from build123d import *

# Parameters (mm, degrees)
SKIZZE2_W                        = 120
SKIZZE2_H                        = 39.364160046
AUFSATZ_LINEAR_AUSTRAGEN1_DEPTH  = 30
SKIZZE24_R                       = 1.55
SCHNITT_LINEAR_AUSTRAGEN4_DEPTH  = 130.805766806
SKIZZE46_R                       = 2.85
SCHNITT_LINEAR_AUSTRAGEN15_DEPTH = 10
SCHNITT_LINEAR_START             = -5
SCHNITT_LINEAR_AUSTRAGEN25_DEPTH = 2.7
LINEARES_MUSTER1_COUNT           = 4
LINEARES_MUSTER1_PITCH           = 20
SPIEGELN2_COPY_1_SKETCH_R        = 2.85
SPIEGELN2_COPY_1_DEPTH           = 10
SPIEGELN2_COPY_2_SKETCH_R        = 2.85
SPIEGELN2_COPY_2_DEPTH           = 10
SPIEGELN2_COPY_3_SKETCH_R        = 2.85
SPIEGELN2_COPY_3_DEPTH           = 10
SPIEGELN2_START                  = -5
SPIEGELN2_COPY_4_DEPTH           = 2.7
SPIEGELN2_COPY_5_DEPTH           = 2.7
SPIEGELN2_COPY_6_DEPTH           = 2.7
SKIZZE51_R                       = 1.55
SCHNITT_LINEAR_AUSTRAGEN26_DEPTH = 130.805766806
SKIZZE75_R                       = 0.75
SCHNITT_LINEAR_AUSTRAGEN28_DEPTH = 10
SKIZZE76_R                       = 2
SCHNITT_LINEAR_AUSTRAGEN29_DEPTH = 6
SKIZZE80_R                       = 0.5
SCHNITT_LINEAR_AUSTRAGEN34_DEPTH = 21
SCHNITT_LINEAR_START_2           = -7.5
SKIZZE81_R                       = 0.5
SCHNITT_LINEAR_AUSTRAGEN36_DEPTH = 5
ABSPALTEN3_START                 = 15
ABSPALTEN3_OUTLINE_W             = 120
ABSPALTEN3_OUTLINE_H             = 39.364160046
ABSPALTEN3_OUTLINE_R             = 1.55
ABSPALTEN3_DEPTH                 = 15


# Read off the part's stored shape, not the designer's step: Abspalten3
with BuildPart() as part:
    # Skizze2 → Aufsatz-Linear austragen1 (new body)
    with BuildSketch(Plane.XY):
        with Locations((60, 19.682080023)):
            Rectangle(SKIZZE2_W, SKIZZE2_H)
    extrude(amount=AUFSATZ_LINEAR_AUSTRAGEN1_DEPTH)

    # Skizze24 → Schnitt-Linear austragen4 (cut, through all)
    with BuildSketch(Plane.XY.offset(30)):
        with Locations((40, 31.364160046)):
            Circle(SKIZZE24_R)
        with Locations((60, 31.364160046)):
            Circle(SKIZZE24_R)
        with Locations((80, 31.364160046)):
            Circle(SKIZZE24_R)
        with Locations((100, 31.364160046)):
            Circle(SKIZZE24_R)
    schnitt_linear_austragen4 = extrude(amount=-SCHNITT_LINEAR_AUSTRAGEN4_DEPTH, mode=Mode.SUBTRACT)

    # Skizze46 → Schnitt-Linear austragen15 (cut)
    with BuildSketch(Plane(origin=(0, 0, 0), x_dir=(-1, 0, 0), z_dir=(0, 0, -1))):
        with Locations((-100, 31.364160046)):
            Circle(SKIZZE46_R)
    schnitt_linear_austragen15 = extrude(amount=-SCHNITT_LINEAR_AUSTRAGEN15_DEPTH, mode=Mode.SUBTRACT)

    # Skizze50 → Schnitt-Linear austragen25 (cut)
    with BuildSketch(Plane.XY.offset(30).offset(SCHNITT_LINEAR_START)):
        Polygon((97.15, 33.009608314), (97.15, 39.364160046), (102.85, 39.364160046), (102.85, 33.009608314), (102.85, 29.718711779), (100, 28.073263512), (97.15, 29.718711779), align=None)
    schnitt_linear_austragen25 = extrude(amount=-SCHNITT_LINEAR_AUSTRAGEN25_DEPTH, mode=Mode.SUBTRACT)

    # Lineares Muster1: Schnitt-Linear austragen15, Schnitt-Linear austragen25 ×4
    with Locations(*[(-i * LINEARES_MUSTER1_PITCH, 0, 0) for i in range(1, LINEARES_MUSTER1_COUNT)]):
        add(schnitt_linear_austragen15, mode=Mode.SUBTRACT)
        add(schnitt_linear_austragen25, mode=Mode.SUBTRACT)

    # Spiegeln2: Schnitt-Linear austragen15, Schnitt-Linear austragen25 across plane
    add(schnitt_linear_austragen15.mirror(Plane.ZX.offset(19.764160046)), mode=Mode.SUBTRACT)
    add(schnitt_linear_austragen25.mirror(Plane.ZX.offset(19.764160046)), mode=Mode.SUBTRACT)

    # Spiegeln2 copy 1 sketch → Spiegeln2 copy 1 (cut)
    with BuildSketch(Plane(origin=(-20, 39.528320093, 0), x_dir=(-1, 0, 0), z_dir=(0, 0, -1))):
        with Locations((-100, -31.364160046)):
            Circle(SPIEGELN2_COPY_1_SKETCH_R)
    extrude(amount=-SPIEGELN2_COPY_1_DEPTH, mode=Mode.SUBTRACT)

    # Spiegeln2 copy 2 sketch → Spiegeln2 copy 2 (cut)
    with BuildSketch(Plane(origin=(-40, 39.528320093, 0), x_dir=(-1, 0, 0), z_dir=(0, 0, -1))):
        with Locations((-100, -31.364160046)):
            Circle(SPIEGELN2_COPY_2_SKETCH_R)
    extrude(amount=-SPIEGELN2_COPY_2_DEPTH, mode=Mode.SUBTRACT)

    # Spiegeln2 copy 3 sketch → Spiegeln2 copy 3 (cut)
    with BuildSketch(Plane(origin=(-60, 39.528320093, 0), x_dir=(-1, 0, 0), z_dir=(0, 0, -1))):
        with Locations((-100, -31.364160046)):
            Circle(SPIEGELN2_COPY_3_SKETCH_R)
    extrude(amount=-SPIEGELN2_COPY_3_DEPTH, mode=Mode.SUBTRACT)

    # Spiegeln2 copy 4 sketch → Spiegeln2 copy 4 (cut)
    with BuildSketch(Plane(origin=(-20, 39.528320093, 30), x_dir=(1, 0, 0), z_dir=(0, 0, 1)).offset(SPIEGELN2_START)):
        Polygon((97.15, -33.009608314), (97.15, -39.364160046), (102.85, -39.364160046), (102.85, -33.009608314), (102.85, -29.718711779), (100, -28.073263512), (97.15, -29.718711779), align=None)
    extrude(amount=-SPIEGELN2_COPY_4_DEPTH, mode=Mode.SUBTRACT)

    # Spiegeln2 copy 5 sketch → Spiegeln2 copy 5 (cut)
    with BuildSketch(Plane(origin=(-40, 39.528320093, 30), x_dir=(1, 0, 0), z_dir=(0, 0, 1)).offset(SPIEGELN2_START)):
        Polygon((97.15, -33.009608314), (97.15, -39.364160046), (102.85, -39.364160046), (102.85, -33.009608314), (102.85, -29.718711779), (100, -28.073263512), (97.15, -29.718711779), align=None)
    extrude(amount=-SPIEGELN2_COPY_5_DEPTH, mode=Mode.SUBTRACT)

    # Spiegeln2 copy 6 sketch → Spiegeln2 copy 6 (cut)
    with BuildSketch(Plane(origin=(-60, 39.528320093, 30), x_dir=(1, 0, 0), z_dir=(0, 0, 1)).offset(SPIEGELN2_START)):
        Polygon((97.15, -33.009608314), (97.15, -39.364160046), (102.85, -39.364160046), (102.85, -33.009608314), (102.85, -29.718711779), (100, -28.073263512), (97.15, -29.718711779), align=None)
    extrude(amount=-SPIEGELN2_COPY_6_DEPTH, mode=Mode.SUBTRACT)

    # Spiegeln3: Schnitt-Linear austragen4 across plane
    add(schnitt_linear_austragen4.mirror(Plane.ZX.offset(19.764160046)), mode=Mode.SUBTRACT)

    # Skizze51 → Schnitt-Linear austragen26 (cut, through all)
    with BuildSketch(Plane.XY.offset(30)):
        with Locations((5, 34.364160046)):
            Circle(SKIZZE51_R)
        with Locations((115, 5)):
            Circle(SKIZZE51_R)
    extrude(amount=-SCHNITT_LINEAR_AUSTRAGEN26_DEPTH, mode=Mode.SUBTRACT)

    # Skizze73 → Schnitt-Rotation5 (revolve, cut)
    with BuildSketch(Plane.XY.offset(15)):
        Polygon((15, 19.764160046), (15, 23.264160046), (20, 23.264160046), (20, 24.264160046), (100, 22.682080023), (100, 21.682080023), (105, 21.682080023), (105, 19.682080023), align=None)
    revolve(axis=Axis((105, 19.682080023, 15), (-0.9999995841280241, 0.0009119998787298228, 0)), mode=Mode.SUBTRACT)

    # Skizze75 → Schnitt-Linear austragen28 (cut)
    with BuildSketch(Plane.XY.offset(30)):
        with Locations((21.598259807, 19.682080023)):
            Circle(SKIZZE75_R)
    extrude(amount=-SCHNITT_LINEAR_AUSTRAGEN28_DEPTH, mode=Mode.SUBTRACT)

    # Skizze76 → Schnitt-Linear austragen29 (cut)
    with BuildSketch(Plane.XY.offset(30)):
        with Locations((21.598259807, 19.682080023)):
            Circle(SKIZZE76_R)
    extrude(amount=-SCHNITT_LINEAR_AUSTRAGEN29_DEPTH, mode=Mode.SUBTRACT)

    # Skizze80 → Schnitt-Linear austragen34 (cut)
    with BuildSketch(Plane(origin=(120, 0, 0), x_dir=(0, 0, -1), z_dir=(1, 0, 0))):
        with Locations((-22.000416524, 19.763714623)):
            Circle(SKIZZE80_R)
    schnitt_linear_austragen34 = extrude(amount=-SCHNITT_LINEAR_AUSTRAGEN34_DEPTH, mode=Mode.SUBTRACT)

    # Skizze81 → Schnitt-Linear austragen36 (cut)
    with BuildSketch(Plane.XY.offset(30).offset(SCHNITT_LINEAR_START_2)):
        with Locations(Location((99, 19.682080023, 0), (0, 0, 7.034090001))):
            Circle(SKIZZE81_R)
    schnitt_linear_austragen36 = extrude(amount=-SCHNITT_LINEAR_AUSTRAGEN36_DEPTH, mode=Mode.SUBTRACT)

    # Spiegeln4: Schnitt-Linear austragen34, Schnitt-Linear austragen36 across plane
    add(schnitt_linear_austragen34.mirror(Plane.XY.offset(15)), mode=Mode.SUBTRACT)
    add(schnitt_linear_austragen36.mirror(Plane.XY.offset(15)), mode=Mode.SUBTRACT)

    # Abspalten3 outline → Abspalten3 (cut)
    with BuildSketch(Plane.XY.offset(ABSPALTEN3_START)):
        with Locations((60, 19.682080023)):
            Rectangle(ABSPALTEN3_OUTLINE_W, ABSPALTEN3_OUTLINE_H)
        with Locations((115, 5)):
            Circle(ABSPALTEN3_OUTLINE_R, mode=Mode.SUBTRACT)
        with Locations((5, 34.364160046)):
            Circle(ABSPALTEN3_OUTLINE_R, mode=Mode.SUBTRACT)
        with Locations((40, 31.364160046)):
            Circle(ABSPALTEN3_OUTLINE_R, mode=Mode.SUBTRACT)
        with Locations((60, 31.364160046)):
            Circle(ABSPALTEN3_OUTLINE_R, mode=Mode.SUBTRACT)
        with Locations((80, 31.364160046)):
            Circle(ABSPALTEN3_OUTLINE_R, mode=Mode.SUBTRACT)
        with Locations((100, 31.364160046)):
            Circle(ABSPALTEN3_OUTLINE_R, mode=Mode.SUBTRACT)
        with Locations((40, 8.164160046)):
            Circle(ABSPALTEN3_OUTLINE_R, mode=Mode.SUBTRACT)
        with Locations((60, 8.164160046)):
            Circle(ABSPALTEN3_OUTLINE_R, mode=Mode.SUBTRACT)
        with Locations((80, 8.164160046)):
            Circle(ABSPALTEN3_OUTLINE_R, mode=Mode.SUBTRACT)
        with Locations((100, 8.164160046)):
            Circle(ABSPALTEN3_OUTLINE_R, mode=Mode.SUBTRACT)
    extrude(amount=ABSPALTEN3_DEPTH, mode=Mode.SUBTRACT)


solid = part.part
The model under review builds one solid part; all positions refer to its coordinate system, in mm. A direction names the side the tool comes from. Round coordinates to 2 decimals unless told otherwise and drop trailing zeros. Order: outer loops, then holes, each group sorted by start corner. A loop starts at its lowest first (then second) coordinate and runs counter-clockwise, first axis right, second up. Notation, with made-up numbers: (-6, 73) -> (5, 73) arc R21 ccw to (5, 98) -> close; hole circle Ø6 at (32.5, 54.5). An arc over 180 degrees is marked (long way). Use CSV: the item, a comma, the result in double quotes. Start each with the question number.
(1) Consider section B-B on z = 3. State how many separate pieces and enclosed holes the cut face has, and give its area (3 significant figures).
(2) Tool access review of faces 1 (the face through (81.48, 7.7, 12.54)), 2 (the face through (105, 20, 14)), 3 (the face through (78.8, 30.1, 10)): name each direction out of +Z, -Z, +X, -X, +Y, -Y from which nothing blocks a thin tool from reaching the whole face with its end or side.
(3) Wall thickness on probe 1 along Y at (x, z) = (40, 4); probe 2 along X at (y, z) = (8.5, 2.5); probe 3 along X at (y, z) = (9, 3.75): over which ranges is each line inside the solid? List them lowest first. Write a range as from..to.
(4) Mouldability with a two-part tool opening along Y and no side actions: class faces 4 (the face through (78.8, 6.9, 10)), 5 (the face through (59, 0, 7)), 6 (the face through (102.26, 29.63, 4.93)) as pulls with the +Y half, pulls with the -Y half, needs draft (parallel to the pull), parting line crosses it, or undercut.
(5) Consider section A-A on x = 5. Write out the cut boundary in (y, z), and give its area (3 significant figures).
(6) Insertion check: pin 1 (4 mm diameter, centred on x = 40, y = 8.16, fed in from -Z); pin 2 (1.9 mm diameter, centred on x = 115, y = 5, fed in from +Z). Each pin has a flat end and moves straight along its axis. Give the tip position at first contact, or say it passes through.
Responses:
1,separate pieces,"1"
1,enclosed holes,"10"
1,area,"4,500 mm²"
2,face 1,"+Z, -Z"
2,face 2,"+Z"
2,face 3,"-Z"
3,probe 1,"0..5.31, 11.01..28.51, 34.21..39.36"
3,probe 2,"0..37.17, 42.83..57.17, 62.83..77.17, 82.83..97.17, 102.83..120"
3,probe 3,"0..37.28, 42.72..57.28, 62.72..77.28, 82.72..97.28, 102.72..120"
4,face 4,"undercut"
4,face 5,"pulls with the -Y half"
4,face 6,"undercut"
5,outline,"(0, 0) -> (32.81, 0) -> (32.81, 15) -> (0, 15) -> close; (35.91, 0) -> (39.36, 0) -> (39.36, 15) -> (35.91, 15) -> close"
5,area,"544 mm²"
6,pin 1,"z = 10"
6,pin 2,"through"
